```python
from build123d import *

# Parameters (mm, degrees)
SKETCH1_R                            = 3.75
BOSS_EXTRUDE1_DEPTH                  = 15
SKETCH2_W                            = 55
SKETCH2_H                            = 5
BOSS_EXTRUDE2_DEPTH                  = 30
F_3_2_3_2_DIAMETER_HOLE1_D           = 3.2
F_3_2_3_2_DIAMETER_HOLE1_CSINK_D     = 3.25
F_3_2_3_2_DIAMETER_HOLE1_CSINK_ANGLE = 90
CHAMFER1_SIZE                        = 4
CUT_EXTRUDE1_DEPTH                   = 146.902364614
CUT_EXTRUDE1_DEPTH_BACK              = 146.902364614
CHAMFER2_SIZE                        = 2.5


with BuildPart() as part:
    # Sketch1 → Boss-Extrude1 (new body)
    with BuildSketch(Plane.XY):
        Polygon((0, 0), (-12.5, 0), (-12.5, 142.5), (12.5, 142.5), (12.5, 0), align=None)
        with Locations((0, 132.5)):
            Circle(SKETCH1_R, mode=Mode.SUBTRACT)
        with Locations((0, 117.5)):
            Circle(SKETCH1_R, mode=Mode.SUBTRACT)
        with Locations((0, 102.5)):
            Circle(SKETCH1_R, mode=Mode.SUBTRACT)
        with Locations((0, 87.5)):
            Circle(SKETCH1_R, mode=Mode.SUBTRACT)
    extrude(amount=BOSS_EXTRUDE1_DEPTH)

    # Sketch2 → Boss-Extrude2 (add)
    with BuildSketch(Plane(origin=(0, 0, 0), x_dir=(-1, 0, 0), z_dir=(0, 0, -1))):
        with Locations((0, 2.5)):
            Rectangle(SKETCH2_W, SKETCH2_H)
    extrude(amount=-BOSS_EXTRUDE2_DEPTH)

    # Ø3.2 (3.2) Diameter Hole1 (through all)
    with Locations(Plane(origin=(0, 5, 0), x_dir=(1, 0, 0), z_dir=(0, 1, 0))):
        with Locations((-22.5, -5), (-22.5, -25), (22.5, -25), (22.5, -5)):
            CounterSinkHole(F_3_2_3_2_DIAMETER_HOLE1_D / 2, F_3_2_3_2_DIAMETER_HOLE1_CSINK_D / 2, counter_sink_angle=F_3_2_3_2_DIAMETER_HOLE1_CSINK_ANGLE)

    # Chamfer1
    chamfer1_edges = [part.edges().sort_by_distance(p)[0] for p in [
        (-12.5, 5, 7.5),
        (0, 5, 15),
        (12.5, 5, 7.5),
    ]]
    chamfer(chamfer1_edges, length=CHAMFER1_SIZE)

    # Sketch6 → Cut-Extrude1 (cut, two sides: drawn at the far end of the back side and taken through both)
    with BuildSketch(Plane.XY.offset(15).offset(-CUT_EXTRUDE1_DEPTH_BACK)):
        with BuildLine():
            ThreePointArc((-8.942906574, 110.830449827), (-11.555147059, 113.720588235), (-12.5, 117.5))
            Line((-12.5, 117.5), (-12.5, 102.5))
            ThreePointArc((-12.5, 102.5), (-11.555147059, 106.279411765), (-8.942906574, 109.169550173))
            ThreePointArc((-8.942906574, 109.169550173), (-8.5, 110), (-8.942906574, 110.830449827))
        make_face()
        with BuildLine():
            Line((12.5, 87.5), (12.5, 102.5))
            ThreePointArc((12.5, 102.5), (11.555147059, 98.720588235), (8.942906574, 95.830449827))
            ThreePointArc((8.942906574, 95.830449827), (8.5, 95), (8.942906574, 94.169550173))
            ThreePointArc((8.942906574, 94.169550173), (11.555147059, 91.279411765), (12.5, 87.5))
        make_face()
        with BuildLine():
            Line((12.5, 102.5), (12.5, 117.5))
            ThreePointArc((12.5, 117.5), (11.555147059, 113.720588235), (8.942906574, 110.830449827))
            ThreePointArc((8.942906574, 110.830449827), (8.5, 110), (8.942906574, 109.169550173))
            ThreePointArc((8.942906574, 109.169550173), (11.555147059, 106.279411765), (12.5, 102.5))
        make_face()
        with BuildLine():
            Line((12.5, 117.5), (12.5, 132.5))
            ThreePointArc((12.5, 132.5), (11.555147059, 128.720588235), (8.942906574, 125.830449827))
            ThreePointArc((8.942906574, 125.830449827), (8.5, 125), (8.942906574, 124.169550173))
            ThreePointArc((8.942906574, 124.169550173), (11.555147059, 121.279411765), (12.5, 117.5))
        make_face()
        with BuildLine():
            Line((12.5, 142.5), (2.5, 142.5))
            ThreePointArc((2.5, 142.5), (9.571067812, 139.571067812), (12.5, 132.5))
            Line((12.5, 132.5), (12.5, 142.5))
        make_face()
        with BuildLine():
            Line((-12.5, 142.5), (-12.5, 132.5))
            ThreePointArc((-12.5, 132.5), (-9.571067812, 139.571067812), (-2.5, 142.5))
            Line((-2.5, 142.5), (-12.5, 142.5))
        make_face()
        with BuildLine():
            ThreePointArc((-8.942906574, 125.830449827), (-11.555147059, 128.720588235), (-12.5, 132.5))
            Line((-12.5, 132.5), (-12.5, 117.5))
            ThreePointArc((-12.5, 117.5), (-11.555147059, 121.279411765), (-8.942906574, 124.169550173))
            ThreePointArc((-8.942906574, 124.169550173), (-8.5, 125), (-8.942906574, 125.830449827))
        make_face()
        with BuildLine():
            Line((-12.5, 102.5), (-12.5, 87.5))
            ThreePointArc((-12.5, 87.5), (-11.555147059, 91.279411765), (-8.942906574, 94.169550173))
            ThreePointArc((-8.942906574, 94.169550173), (-8.5, 95), (-8.942906574, 95.830449827))
            ThreePointArc((-8.942906574, 95.830449827), (-11.555147059, 98.720588235), (-12.5, 102.5))
        make_face()
    extrude(amount=CUT_EXTRUDE1_DEPTH + CUT_EXTRUDE1_DEPTH_BACK, mode=Mode.SUBTRACT)

    # Chamfer2
    chamfer2_edges = [part.edges().sort_by_distance(p)[0] for p in [
        (-3.75, 117.5, 15),
        (-3.75, 102.5, 15),
        (-3.75, 132.5, 15),
        (-3.75, 87.5, 15),
    ]]
    chamfer(chamfer2_edges, length=CHAMFER2_SIZE)


solid = part.part
```
CAD build for the part. Positions are in the model's coordinates, mm. A direction names the side the tool comes from. Round coordinates to 2 decimals unless told otherwise and drop trailing zeros. Write each loop counter-clockwise with the first axis right and the second up, starting at its lowest first coordinate (ties: lowest second). Pieces come first, ordered by that corner, then holes. Notation, with made-up numbers: (26, 59.25) - (84, 59.25) arc R27 ccw to (84, 84.25) - close; hole circle Ø8 at (14.5, -11.75). An arc over 180 degrees is marked (long way). Return JSON: item names as keys, results as strings. Group by question number.
Item 1: Band-saw the part on D-D on y = 50.5. List the corners of the cut face in (x, z).
Item 2: Band-saw the part on B-B on x = 0. State how many separate pieces and enclosed holes the cut face has, plus the area to 3 significant figures.
Item 3: 3-axis set-ups, long thin cutter, end or side, ignore diameter. For faces 1 (the face through (0, 5, 21)), 2 (the face through (11.58, 128.77, 7.4)), 3 (the face through (-12.5, 48, 7)): which of +Z, -Z, +X, -X, +Y, -Y reach the whole face in a straight line?
Item 4: Band-saw the part on A-A on x = 22.5. List the corners of the cut face in (y, z) (3 decimals).
Item 5: Band-saw the part on C-C on z = 25. List the corners of the cut face in (x, y) (3 decimals), plus the area to 3 significant figures.
Item 6: Mould opens along Z. For faces 4 (the face through (0, 142.5, 7)), 5 (the face through (1.8, 129.03, 12.66)), 6 (the face through (-6, 72, 0)), 7 (the face through (-24.026, 2.453, 4.519)) say: +Z half, -Z half, draft (parallel to the pull), parting line (faces both ways), or undercut.
Item 7: Probe probe 1 along Y at (x, z) = (0, 5.5); probe 2 along X at (y, z) = (3.55, 25); probe 3 along Z at (x, y) = (-22.5, 2.5). List the from-to ranges inside material, lowest first.
Item 8: Flat gauge pins, fed straight in: pin 1 Ø6 at (x, z) = (8.5, 7) entering from +Y; pin 2 Ø3 at (x, z) = (-11.5, 25) entering from +Y; pin 3 Ø4.5 at (y, z) = (41.5, 5.5) entering from -X. Where does each tip first touch, or does it go through?
Resolved:
{
 "1": {"outline": "(-12.5, 0) - (12.5, 0) - (12.5, 15) - (-12.5, 15) - close"},
 "2": {"separate pieces": "5", "enclosed holes": "0", "area": "1,750 mm²"},
 "3": {"face 1": "+Z, +Y", "face 2": "+Z, -Z, +X", "face 3": "+Z, -Z, -X, +Y"},
 "4": {"outline": "(0, 0) - (5, 0) - (5, 3.375) - (4.975, 3.4) - (0, 3.4) - close; (0, 6.6) - (4.975, 6.6) - (5, 6.625) - (5, 23.375) - (4.975, 23.4) - (0, 23.4) - close; (0, 26.6) - (4.975, 26.6) - (5, 26.625) - (5, 30) - (0, 30) - close"},
 "5": {"outline": "(-27.5, 0) - (-24.1, 0) - (-24.1, 4.975) - (-24.125, 5) - (-27.5, 5) - close; (-20.9, 0) - (20.9, 0) - (20.9, 4.975) - (20.875, 5) - (-20.875, 5) - (-20.9, 4.975) - close; (24.1, 0) - (27.5, 0) - (27.5, 5) - (24.125, 5) - (24.1, 4.975) - close", "area": "243 mm²"},
 "6": {"face 4": "draft", "face 5": "+Z half", "face 6": "-Z half", "face 7": "undercut"},
 "7": {"probe 1": "y = 0 to 83.75, 91.25 to 98.75, 106.25 to 113.75, 121.25 to 128.75, 136.25 to 142.5", "probe 2": "x = -27.5 to -24.1, -20.9 to 20.9, 24.1 to 27.5", "probe 3": "z = 0 to 3.4, 6.6 to 23.4, 26.6 to 30"},
 "8": {"pin 1": "stops at y = 142.04", "pin 2": "stops at y = 5", "pin 3": "stops at x = -12.5"}
}
